```python
from build123d import *

# Parameters (mm, degrees)
SKETCH002_R     = 1.6
PAD002_DEPTH    = 4
SKETCH007_W     = 32
SKETCH007_H     = 36
SKETCH007_W_2   = 24
SKETCH007_H_2   = 28
PAD006_DEPTH    = 10
SKETCH008_R     = 1.6
POCKET_DEPTH    = 46.001
SKETCH020_W     = 32
SKETCH020_H     = 4
PAD015_DEPTH    = 32
SKETCH021_R     = 10.5
POCKET004_DEPTH = 5


with BuildPart() as part:
    # Sketch002 → Pad002 (new body)
    with BuildSketch(Plane.XZ):
        with BuildLine():
            Line((-29, 50), (29, 50))
            ThreePointArc((30, 49), (29.707107, 49.707107), (29, 50))
            Line((30, 49), (30, -9))
            ThreePointArc((29, -10), (29.707107, -9.707107), (30, -9))
            Line((29, -10), (-29, -10))
            ThreePointArc((-30, -9), (-29.707107, -9.707107), (-29, -10))
            Line((-30, -9), (-30, 49))
            ThreePointArc((-29, 50), (-29.707107, 49.707107), (-30, 49))
        make_face()
        with Locations((-25, -5)):
            Circle(SKETCH002_R, mode=Mode.SUBTRACT)
        with Locations((-25, 45)):
            Circle(SKETCH002_R, mode=Mode.SUBTRACT)
        with Locations((25, 45)):
            Circle(SKETCH002_R, mode=Mode.SUBTRACT)
        with Locations((25, -5)):
            Circle(SKETCH002_R, mode=Mode.SUBTRACT)
    extrude(amount=-PAD002_DEPTH)

    # Sketch007 (on Face13 of Pad002) → Pad006 (join)
    with BuildSketch(Plane.XZ):
        with Locations((0, 22)):
            Rectangle(SKETCH007_W, SKETCH007_H)
        with Locations((0, 22)):
            Rectangle(SKETCH007_W_2, SKETCH007_H_2, mode=Mode.SUBTRACT)
    extrude(amount=PAD006_DEPTH)

    # Sketch008 (on Face17 of Pad006) → Pocket (cut, through all)
    with BuildSketch(Plane(origin=(-16, 0, 0), x_dir=(0, 0, -1), z_dir=(-1, 0, 0))):
        with Locations((-32, 5)):
            Circle(SKETCH008_R)
        with Locations((-12, 5)):
            Circle(SKETCH008_R)
    extrude(amount=-POCKET_DEPTH, mode=Mode.SUBTRACT)

    # Sketch020 (on Face19 of Pocket) → Pad015 (join)
    with BuildSketch(Plane.XZ.offset(10)):
        with Locations((0, 38)):
            Rectangle(SKETCH020_W, SKETCH020_H)
    extrude(amount=PAD015_DEPTH)

    # Sketch021 (on Face19 of Pad015) → Pocket004 (cut)
    with BuildSketch(Plane(origin=(0, 0, 40), x_dir=(-1, 0, 0), z_dir=(0, 0, 1))):
        with Locations((0, 26)):
            Circle(SKETCH021_R)
    extrude(amount=-POCKET004_DEPTH, mode=Mode.SUBTRACT)


solid = part.part
```
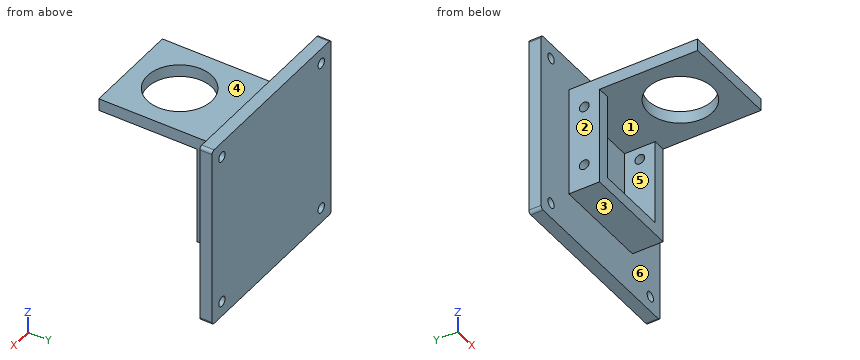
Geometry check sheet. Reference: the model listing, model coordinates, mm. Face numbers are marked on the shaded views. A direction names the side the tool comes from. Round coordinates to 2 decimals unless told otherwise and drop trailing zeros. Loops run counter-clockwise (first coordinate to the right, second up) from the corner with the lowest first, then second, coordinate; pieces in that order, holes last. Notation, with made-up numbers: (-18.5, 47.5) - (16.5, 47.5) arc R16 cw to (16.5, 70.5) - close; hole circle Ø7 at (-23.75, 12). An arc over 180 degrees is marked (long way). Use a Markdown table: item, result.
Q1. Cross-section at B-B on z = 45. Record the cut outline in (x, y).
Solutions:
| item | result |
|---|---|
| outline | (-30, 0) - (-26.6, 0) - (-26.6, 4) - (-30, 4) - close; (-23.4, 0) - (23.4, 0) - (23.4, 4) - (-23.4, 4) - close; (26.6, 0) - (30, 0) - (30, 4) - (26.6, 4) - close |
Q2. Go/stop test with flat-tipped pins: P1, Ø8, axis at x = -8.5, y = -21, coming from the -Z side; P2, Ø5, axis at y = -5, z = 12, coming from the +X side; P3, Ø1.9, axis at y = -5, z = 32, coming from the -X side; P4, Ø9.5, axis at x = -6.5, z = 24.5, coming from the -Y side. Record where each tip stops, or that it passes through.
Solutions:
| item | result |
|---|---|
| P1 | stops at z = 36 |
| P2 | stops at x = 16 |
| P3 | passes through |
| P4 | stops at y = 0 |
Q3. Draft check along Z on the marked faces 4, 5 and 6. Enter one of: released by +Z, released by -Z, zero draft, split by the parting line, or undercut.
Solutions:
| item | result |
|---|---|
| face 4 | released by +Z |
| face 5 | undercut |
| face 6 | zero draft |
Q4. Access from +Z, -Z, +X, -X, +Y, -Y to the whole of each face (thin tool, end or side, straight path). Record for the marked faces 1, 2 and 3.
Solutions:
| item | result |
|---|---|
| face 1 | -Y |
| face 2 | +Z, -Z, -X, -Y |
| face 3 | -Z, +X, -X, -Y |
Q5. Material ranges on line 1 (Z direction, x = -25, y = 2.3); line 2 (Z direction, x = 13.2, y = -5); line 3 (Y direction, x = 0, z = 37.7), recorded low to high.
Solutions:
| item | result |
|---|---|
| line 1 | z = -10 to -6.6, -3.4 to 43.4, 46.6 to 50 |
| line 2 | z = 4 to 10.4, 13.6 to 30.4, 33.6 to 40 |
| line 3 | y = -42 to -36.5, -15.5 to 4 |
Q6. Cross-section at D-D on x = -25. Record the cut outline in (y, z), plus the area to 3 significant figures.
Solutions:
| item | result |
|---|---|
| outline | (0, -10) - (4, -10) - (4, -6.6) - (0, -6.6) - close; (0, -3.4) - (4, -3.4) - (4, 43.4) - (0, 43.4) - close; (0, 46.6) - (4, 46.6) - (4, 50) - (0, 50) - close |
| area | 214 mm2 |
Q7. Cross-section at A-A on x = -14.5. Record the cut outline in (y, z).
Solutions:
| item | result |
|---|---|
| outline | (-42, 36) - (-10, 36) - (-10, 4) - (0, 4) - (0, -10) - (4, -10) - (4, 50) - (0, 50) - (0, 40) - (-42, 40) - close; hole circle Ø3.2 at (-5, 12); hole circle Ø3.2 at (-5, 32) |
Q8. Cross-section at C-C on y = -1. Record the cut outline in (x, z).
Solutions:
| item | result |
|---|---|
| outline | (-16, 4) - (16, 4) - (16, 40) - (-16, 40) - close; hole (-12, 8) - (12, 8) - (12, 36) - (-12, 36) - close |
